Could you check a few things on this model? Use its own coordinates, in mm. Round coordinates to 2 decimals unless told otherwise and drop trailing zeros. Loops run counter-clockwise (first coordinate to the right, second up) from the corner with the lowest first, then second, coordinate; pieces in that order, holes last. Notation, with made-up numbers: (9.5, 53.25) -> (45.5, 53.25) arc R22 cw to (45.5, 80.25) -> close; hole circle Ø1 at (-40, -19). An arc over 180 degrees is marked (long way). Write each question's results on one line, items separated by ' | '.
from build123d import *

# Parameters (mm, degrees)
STOCK_NOS_TANK_PLATE_SUPPORT_VALVE_1_ANGLE = 180
SKETCH4_R                                  = 3.175
CUT_EXTRUDE2_DEPTH                         = 60.198


# Read off the part's stored shape, not the designer's step: Stock-Nos Tank Plate Support Valve-1
with BuildPart() as part:
    # Stock-Nos Tank Plate Support Valve-1 out → Stock-Nos Tank Plate Support Valve-1 (revolve)
    with BuildSketch(Plane(origin=(0, 0, 0), x_dir=(0, 0, -1), z_dir=(1, 0, 0))):
        Polygon((83.82, 6.35), (56.67515342, 6.35), (31.75, -6.35), (83.82, -6.35), align=None)
    revolve(axis=Axis((0, 0, 0), (0, 1, 0)), revolution_arc=STOCK_NOS_TANK_PLATE_SUPPORT_VALVE_1_ANGLE)

    # Sketch4 → Cut-Extrude2 (cut)
    with BuildSketch(Plane(origin=(0, 0, 0), x_dir=(0, 0, -1), z_dir=(1, 0, 0))):
        with Locations((-68.035369102, 0)):
            Circle(SKETCH4_R)
    cut_extrude2 = extrude(amount=-CUT_EXTRUDE2_DEPTH, mode=Mode.SUBTRACT)

    # Mirror1: Cut-Extrude2 across plane
    add(cut_extrude2.mirror(Plane.XY), mode=Mode.SUBTRACT)


solid = part.part
1) I'm going to push flat-ended pins straight in: pin 1 (1.5 mm diameter, centred on x = -24.5, y = 3.5, fed in from -Z); pin 2 (3 mm diameter, centred on x = -28, y = -3.5, fed in from +Z); pin 3 (4 mm diameter, centred on y = 0, z = -68.04, fed in from +X); pin 4 (4 mm diameter, centred on y = -1.5, z = -11, fed in from +X). Where does each tip first touch, or does it pass through?
Model answer:
pin 1: stops at z = -80.38 | pin 2: stops at z = 79.52 | pin 3: passes through | pin 4: stops at x = -35.64
2) I want a section at B-B, the plane x = -16. Give the number of separate pieces and of enclosed holes in the cut face, plus the area to 3 significant figures.
Model answer:
separate pieces: 2 | enclosed holes: 2 | area: 982 mm2
3) I need wall thicknesses on line 1 (Y direction, x = -36.5, z = -66.5); line 2 (Z direction, x = -20.5, y = -2); line 3 (Z direction, x = -30, y = 5). Which ranges of each line are inside material? Lowest first, please.
Model answer:
line 1: y = -6.35 to -2.78, 2.78 to 6.35 | line 2: z = -81.27 to -70.5, -65.57 to -34.68, 34.68 to 65.57, 70.5 to 81.27 | line 3: z = -78.27 to -44.93, 44.93 to 78.27
4) I want a section at D-D, the plane x = -65. Write out the boundary of the cut face in (y, z), plus the area to 3 significant figures.
Model answer:
outline: (-6.35, -52.92) -> (6.35, -52.92) -> (6.35, 52.92) -> (-6.35, 52.92) -> close | area: 1,340 mm2
5) I want a section at C-C, the plane z = 0. Write out the boundary of the cut face in (x, y).
Model answer:
outline: (-83.82, -6.35) -> (-31.75, -6.35) -> (-56.68, 6.35) -> (-83.82, 6.35) -> close
6) I want a section at A-A, the plane y = 0. Write out the boundary of the cut face in (x, z), plus the area to 3 significant figures.
Model answer:
outline: (-53.09, -64.86) -> (0, -64.86) -> (0, -44.21) arc R44.21 cw to (0, 44.21) -> (0, 64.86) -> (-53.09, 64.86) arc R83.82 ccw to start; (-44.21, -71.21) arc R83.82 ccw to (0, -83.82) -> (0, -71.21) -> close; (-44.21, 71.21) -> (0, 71.21) -> (0, 83.82) arc R83.82 ccw to start | area: 7,350 mm2
7) If we mould it in two halves opening along Z, with no side actions, what happens to faces 1 (the conical face through (-32.952, -5.733, -0.725)), 2 (the flat face through (-42, -6.35, -1)), 3 (the cylindrical face through (-83.8, 0.1, -1.8))? For each: released by +Z, released by -Z, zero draft, split by the parting line, or undercut.
Model answer:
face 1: undercut | face 2: zero draft | face 3: split by the parting line
